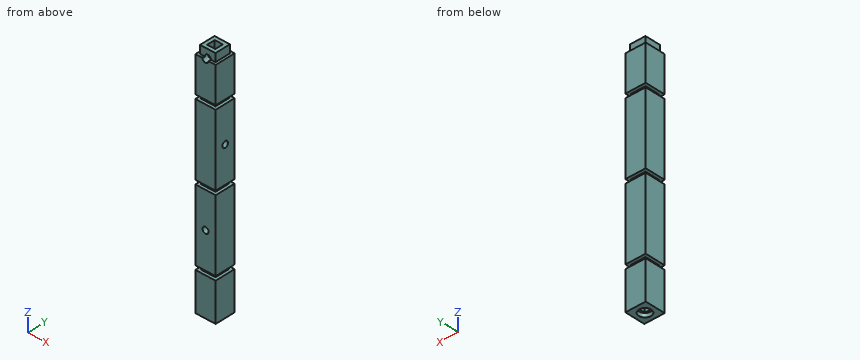
from build123d import *

# Parameters (mm, degrees)
F0_W      = 31.75
F0_H      = 31.75
F1_DEPTH  = 60.33
F2_W      = 22.23
F2_H      = 22.23
F3_DEPTH  = 6.35
F4_W      = 31.75
F4_H      = 31.75
F5_DEPTH  = 112.71
F6_W      = 22.23
F6_H      = 22.23
F7_DEPTH  = 6.35
F8_W      = 31.75
F8_H      = 31.75
F8_W_2    = 22.23
F8_H_2    = 22.23
F9_DEPTH  = 112.71
F10_W     = 22.23
F10_H     = 22.23
F11_DEPTH = 6.35
F12_W     = 31.75
F12_H     = 31.75
F12_W_2   = 22.23
F12_H_2   = 22.23
F13_DEPTH = 112.71
F14_W     = 22.23
F14_H     = 22.23
F15_DEPTH = 6.35
F16_W     = 31.75
F16_H     = 31.75
F17_DEPTH = 112.71
F18_W     = 22.23
F18_H     = 22.23
F19_DEPTH = 6.35
F20_W     = 31.75
F20_H     = 31.75
F20_W_2   = 22.23
F20_H_2   = 22.23
F21_DEPTH = 112.71
F22_W     = 22.23
F22_H     = 22.23
F23_DEPTH = 6.35
F24_W     = 31.75
F24_H     = 31.75
F24_W_2   = 22.23
F24_H_2   = 22.23
F25_DEPTH = 25.4
F26_W     = 22.23
F26_H     = 22.23
F27_DEPTH = 6.35
F28_W     = 31.75
F28_H     = 31.75
F28_W_2   = 22.23
F28_H_2   = 22.23
F29_DEPTH = 31.75
F32_DEPTH = 12.7
F34_DEPTH = 12.7
F36_DEPTH = 12.7
F38_DEPTH = 12.7
F40_DEPTH = 12.7
F41_W     = 12.7
F41_H     = 12.7
F42_DEPTH = 736.6
F43_DEPTH = 6.35
F44_W     = 31.75
F44_H     = 351.79
F45_DEPTH = 76.2
F46_W     = 31.75
F46_H     = 31.75
F46_W_2   = 24.13
F46_H_2   = 24.13
F47_DEPTH = 12.7


with BuildPart() as f1:
    # F0 (on Top) → F1 (new body)
    with BuildSketch(Plane.XY):
        with Locations((15.875, 15.875)):
            Rectangle(F0_W, F0_H)
    extrude(amount=F1_DEPTH)

    # F2 (on face) → F3 (join)
    with BuildSketch(Plane.XY.offset(60.33)):
        with Locations((15.875, 15.875)):
            Rectangle(F2_W, F2_H)
    extrude(amount=F3_DEPTH)

    # F4 (on face) → F5 (join)
    with BuildSketch(Plane.XY.offset(66.68)):
        with Locations((15.875, 15.875)):
            Rectangle(F4_W, F4_H)
    extrude(amount=F5_DEPTH)

    # F6 (on face) → F7 (join)
    with BuildSketch(Plane.XY.offset(179.39)):
        with Locations((15.875, 15.875)):
            Rectangle(F6_W, F6_H)
    extrude(amount=F7_DEPTH)

    # F8 (on face) → F9 (join)
    with BuildSketch(Plane.XY.offset(185.74)):
        with Locations((15.875, 15.875)):
            Rectangle(F8_W, F8_H)
        with Locations((15.875, 15.875)):
            Rectangle(F8_W_2, F8_H_2, mode=Mode.SUBTRACT)
        with Locations((15.875, 15.875)):
            Rectangle(F8_W_2, F8_H_2)
    extrude(amount=F9_DEPTH)

    # F10 (on face) → F11 (join)
    with BuildSketch(Plane.XY.offset(298.45)):
        with Locations((15.875, 15.875)):
            Rectangle(F10_W, F10_H)
    extrude(amount=F11_DEPTH)

    # F12 (on face) → F13 (join)
    with BuildSketch(Plane.XY.offset(304.8)):
        with Locations((15.875, 15.875)):
            Rectangle(F12_W, F12_H)
        with Locations((15.875, 15.875)):
            Rectangle(F12_W_2, F12_H_2, mode=Mode.SUBTRACT)
        with Locations((15.875, 15.875)):
            Rectangle(F12_W_2, F12_H_2)
    extrude(amount=F13_DEPTH)

    # F14 (on face) → F15 (join)
    with BuildSketch(Plane.XY.offset(417.51)):
        with Locations((15.875, 15.875)):
            Rectangle(F14_W, F14_H)
    extrude(amount=F15_DEPTH)

    # F16 (on face) → F17 (join)
    with BuildSketch(Plane.XY.offset(423.86)):
        with Locations((15.875, 15.875)):
            Rectangle(F16_W, F16_H)
    extrude(amount=F17_DEPTH)

    # F18 (on face) → F19 (join)
    with BuildSketch(Plane.XY.offset(536.57)):
        with Locations((15.875, 15.875)):
            Rectangle(F18_W, F18_H)
    extrude(amount=F19_DEPTH)

    # F20 (on face) → F21 (join)
    with BuildSketch(Plane.XY.offset(542.92)):
        with Locations((15.875, 15.875)):
            Rectangle(F20_W, F20_H)
        with Locations((15.875, 15.875)):
            Rectangle(F20_W_2, F20_H_2, mode=Mode.SUBTRACT)
        with Locations((15.875, 15.875)):
            Rectangle(F20_W_2, F20_H_2)
    extrude(amount=F21_DEPTH)

    # F22 (on face) → F23 (join)
    with BuildSketch(Plane.XY.offset(655.63)):
        with Locations((15.875, 15.875)):
            Rectangle(F22_W, F22_H)
    extrude(amount=F23_DEPTH)

    # F24 (on face) → F25 (join)
    with BuildSketch(Plane.XY.offset(661.98)):
        with Locations((15.875, 15.875)):
            Rectangle(F24_W, F24_H)
        with Locations((15.875, 15.875)):
            Rectangle(F24_W_2, F24_H_2, mode=Mode.SUBTRACT)
        with Locations((15.875, 15.875)):
            Rectangle(F24_W_2, F24_H_2)
    extrude(amount=F25_DEPTH)

    # F26 (on face) → F27 (join)
    with BuildSketch(Plane.XY.offset(687.38)):
        with Locations((15.875, 15.875)):
            Rectangle(F26_W, F26_H)
    extrude(amount=F27_DEPTH)

    # F28 (on face) → F29 (join)
    with BuildSketch(Plane.XY.offset(693.73)):
        with Locations((15.875, 15.875)):
            Rectangle(F28_W, F28_H)
        with Locations((15.875, 15.875)):
            Rectangle(F28_W_2, F28_H_2, mode=Mode.SUBTRACT)
        with Locations((15.875, 15.875)):
            Rectangle(F28_W_2, F28_H_2)
    extrude(amount=F29_DEPTH)

    # F31 (on face) → F32 (cut)
    with BuildSketch(Plane.XZ):
        with BuildLine():
            Line((15.875, 123.035), (20.64, 123.035))
            ThreePointArc((20.64, 123.035), (12.5056361876, 126.4043638124), (15.875, 118.27))
            Line((15.875, 118.27), (15.875, 123.035))
        make_face()
        with BuildLine():
            ThreePointArc((15.875, 118.27), (19.2443638124, 119.6656361876), (20.64, 123.035))
            Line((20.64, 123.035), (15.875, 123.035))
            Line((15.875, 123.035), (15.875, 118.27))
        make_face()
    extrude(amount=-F32_DEPTH, mode=Mode.SUBTRACT)

    # F33 (on face) → F34 (cut)
    with BuildSketch(Plane.YZ.offset(31.75)):
        with BuildLine():
            Line((15.875, 242.095), (20.64, 242.095))
            ThreePointArc((20.64, 242.095), (12.5056361876, 245.4643638124), (15.875, 237.33))
            Line((15.875, 237.33), (15.875, 242.095))
        make_face()
        with BuildLine():
            ThreePointArc((15.875, 237.33), (19.2443638124, 238.7256361876), (20.64, 242.095))
            Line((20.64, 242.095), (15.875, 242.095))
            Line((15.875, 242.095), (15.875, 237.33))
        make_face()
    extrude(amount=-F34_DEPTH, mode=Mode.SUBTRACT)

    # F35 (on face) → F36 (cut)
    with BuildSketch(Plane.XZ):
        with BuildLine():
            Line((15.875, 361.155), (20.64, 361.155))
            ThreePointArc((20.64, 361.155), (12.5056361876, 364.5243638124), (15.875, 356.39))
            Line((15.875, 356.39), (15.875, 361.155))
        make_face()
        with BuildLine():
            ThreePointArc((15.875, 356.39), (19.2443638124, 357.7856361876), (20.64, 361.155))
            Line((20.64, 361.155), (15.875, 361.155))
            Line((15.875, 361.155), (15.875, 356.39))
        make_face()
    extrude(amount=-F36_DEPTH, mode=Mode.SUBTRACT)

    # F37 (on face) → F38 (cut)
    with BuildSketch(Plane.YZ.offset(31.75)):
        with BuildLine():
            Line((15.875, 480.215), (20.64, 480.215))
            ThreePointArc((20.64, 480.215), (12.5056361876, 483.5843638124), (15.875, 475.45))
            Line((15.875, 475.45), (15.875, 480.215))
        make_face()
        with BuildLine():
            ThreePointArc((15.875, 475.45), (19.2443638124, 476.8456361876), (20.64, 480.215))
            Line((20.64, 480.215), (15.875, 480.215))
            Line((15.875, 480.215), (15.875, 475.45))
        make_face()
    extrude(amount=-F38_DEPTH, mode=Mode.SUBTRACT)

    # F39 (on face) → F40 (cut)
    with BuildSketch(Plane.XZ):
        with BuildLine():
            Line((15.875, 599.275), (20.64, 599.275))
            ThreePointArc((20.64, 599.275), (12.5056361876, 602.6443638124), (15.875, 594.51))
            Line((15.875, 594.51), (15.875, 599.275))
        make_face()
        with BuildLine():
            ThreePointArc((15.875, 594.51), (19.2443638124, 595.9056361876), (20.64, 599.275))
            Line((20.64, 599.275), (15.875, 599.275))
            Line((15.875, 599.275), (15.875, 594.51))
        make_face()
    extrude(amount=-F40_DEPTH, mode=Mode.SUBTRACT)

    # F41 (on face) → F42 (cut)
    with BuildSketch(Plane.XY.offset(725.48)):
        with Locations((15.87, 15.87)):
            Rectangle(F41_W, F41_H)
    extrude(amount=-F42_DEPTH, mode=Mode.SUBTRACT)

    # F30 (on face) → F43 (cut)
    with BuildSketch(Plane(origin=(0, 0, 0), x_dir=(1, 0, 0), z_dir=(0, 0, -1))):
        with BuildLine():
            ThreePointArc((6.35, -15.875), (9.1398079092, -22.6101920908), (15.875, -25.4))
            Line((15.875, -25.4), (15.875, -15.875))
            Line((15.875, -15.875), (6.35, -15.875))
        make_face()
        with BuildLine():
            Line((15.875, -15.875), (15.875, -25.4))
            ThreePointArc((15.875, -25.4), (22.6101920908, -22.6101920908), (25.4, -15.875))
            ThreePointArc((25.4, -15.875), (15.875, -6.35), (6.35, -15.875))
            Line((6.35, -15.875), (15.875, -15.875))
        make_face()
    extrude(amount=-F43_DEPTH, mode=Mode.SUBTRACT)

    # F44 (on face) → F45 (cut)
    with BuildSketch(Plane.XZ):
        with Locations((15.875, 549.585)):
            Rectangle(F44_W, F44_H)
    extrude(amount=-F45_DEPTH, mode=Mode.SUBTRACT)

    # F46 (on face) → F47 (cut)
    with BuildSketch(Plane.XY.offset(373.69)):
        with Locations((15.875, 15.875)):
            Rectangle(F46_W, F46_H)
        with Locations((15.875, 15.875)):
            Rectangle(F46_W_2, F46_H_2, mode=Mode.SUBTRACT)
    extrude(amount=-F47_DEPTH, mode=Mode.SUBTRACT)


solid = f1.part
Can you work these out from the model? Positions are in its coordinate system, mm. Give positions to 0.01 mm unless a question says otherwise; leave off trailing zeros. Loops run counter-clockwise (first coordinate to the right, second up) from the corner with the lowest first, then second, coordinate; pieces in that order, holes last. Notation, with made-up numbers: (-27.5, -24) - (-23.5, -24) arc R30 ccw to (-23.5, 12) - close; hole circle Ø8 at (0, 23). An arc over 180 degrees is marked (long way). Answer as a JSON object with one key per item and string values.
Q1. If I drill on L1, parallel to Z at x = 1.5, y = 18; L2, parallel to Z at x = 5, y = 4; L3, parallel to Y at x = 21, z = 137, over which ranges is the centre line in solid material (lowest first)?
Geometry says:
{"L1": "0 to 60.33, 66.68 to 179.39, 185.74 to 298.45, 304.8 to 360.99", "L2": "0 to 60.33, 66.68 to 179.39, 185.74 to 298.45, 304.8 to 373.69", "L3": "0 to 9.52, 22.22 to 31.75"}
Q2. Imagine slicing it at A-A on z = 38.5. Write out the boundary of the cut face in (x, y).
Geometry says:
{"outline": "(0, 0) - (31.75, 0) - (31.75, 31.75) - (0, 31.75) - close; hole (9.52, 9.52) - (22.22, 9.52) - (22.22, 22.22) - (9.52, 22.22) - close"}
Q3. Will these pins go through, and if not, where does the flat tip stop? P1, Ø15, axis at x = 20, y = 16, coming from the -Z side; P2, Ø1.9, axis at y = 15, z = 64, coming from the -X side; P3, Ø10, axis at y = 11, z = 367, coming from the -X side.
Geometry says:
{"P1": "z = 0", "P2": "x = 4.76", "P3": "x = 3.81"}
